Geometry: final body of the model. Coordinates: model frame, mm. Coordinates: 2 decimals unless noted, no trailing zeros. Write each loop counter-clockwise with the first axis right and the second up, starting at its lowest first coordinate (ties: lowest second). Pieces come first, ordered by that corner, then holes.
Autodesk Inventor part; units mm, degrees
ref_plane "YZ Plane" through (0, 0, 0) normal (1, 0, 0) x (0, 1, 0)
ref_plane "XZ Plane" through (0, 0, 0) normal (0, 1, 0) x (-1, 0, 0)
ref_plane "XY Plane" through (0, 0, 0) normal (0, 0, 1) x (1, 0, 0)
sketch "スケッチ1" plane through (0, 0, 0) normal (1, 0, 0) x (0, 1, 0)
  circle A0 centre (0, 0) radius 12
  line L0 (12, 0) -> (-12, 0)
  line L1 (-12, 0) -> (-12, -70)
  line L2 (-12, -70) -> (12, -70)
  line L3 (12, -70) -> (12, 0)
  line L4 (-12, -70) -> (-42, -70)
  line L5 (-42, -70) -> (-42, -46)
  line L6 (-42, -46) -> (-12, -46)
  line L7 (-12, -46) -> (-12, -70)
  point P0 (-12, -46)
  dimension "d0" = 24
  dimension "d1" = 70
  dimension "d4" = 24
  dimension "d5" = 30
extrude "押し出し1" add sketch "スケッチ1" along normal blind 5
fillet "フィレット1" radius 20 1 edges at (2.5, -12, -46)
fillet "フィレット3" radius 40 1 edges at (2.5, 12, -70)
fillet "フィレット2" radius 12 2 edges at (2.5, -42, -46) (2.5, -42, -70)
sketch "スケッチ2" plane through (5, 0, 0) normal (1, 0, 0) x (0, 0, -1)
  circle A0 centre (0, 0) radius 8.5
  point P0 (0, 8.5)
  dimension "d8" = 17
hole "穴1" at (5, 8.5, 0) direction (-1, 0, 0) diameter 3.4 end through all
pattern_circular "円形状パターン1" count 4 over 360 about axis through (0, 0, 0) along (1, 0, 0) of "穴1"
fillet "フィレット4" radius 1 16 edges at (5, -29, -70) (5, -38.4853, -66.4853) (5, -42, -57.9687) (5, -38.7464, -49.7216) (5, -12, -13) (5, 0, 12) (5, 12, -15) (5, 0.2843, -58.2843) (0, 12, -15) (0, 0, 12) (0, -12, -13) (0, -38.7464, -49.7216) (0, -42, -57.9687) (0, -38.4853, -66.4853) (0, -29, -70) (0, 0.2843, -58.2843)
properties part number "base9"
Item 1: Material intervals for probe 1 along Y at (x, z) = (1.9, 0); probe 2 along Z at (x, y) = (4.55, 0); probe 3 along Z at (x, y) = (2.55, 8.5), sorted ascending.
Derived:
probe 1: y = -12 to -10.2, -6.8 to 6.8, 10.2 to 12
probe 2: z = -58.33 to -10.2, -6.8 to 6.8, 10.2 to 11.84
probe 3: z = -46.36 to -1.7, 1.7 to 8.47
Item 2: Section A-A, the plane z = -8.5. Output: boundary loops of the cut face in (x, y).
Derived:
outline: (0, -11) arc R1 ccw to (1, -12) - (4, -12) arc R1 ccw to (5, -11) - (5, -1.7) - (0, -1.7) - close; (0, 1.7) - (5, 1.7) - (5, 11) arc R1 ccw to (4, 12) - (1, 12) arc R1 ccw to (0, 11) - close
Item 3: Section B-B, the plane x = 2.75. State how many separate pieces and enclosed holes the cut face has, plus the area to 3 significant figures.
Derived:
separate pieces: 1
enclosed holes: 4
area: 2,270 mm2
Item 4: Pin query (flat end, axial travel): pin 1 (1 mm diameter, centred on x = 4.5, y = -24.5, fed in from -Z); pin 2 (3 mm diameter, centred on x = 1.5, y = -29, fed in from +Z); pin 3 (1 mm diameter, centred on x = 2.5, y = -27.5, fed in from +Z); pin 4 (4.5 mm diameter, centred on y = 8.5, z = 0, fed in from -X). Return the tip coordinate at first contact, or that it passes through.
Derived:
pin 1: stops at z = -69.87
pin 2: stops at z = -45.49
pin 3: stops at z = -45.36
pin 4: stops at x = 0
Item 5: Pull-direction query (Y, two-part tool) for faces 1 (the flat face through (0, -10, -37)), 2 (the flat face through (2, -12, -13)), 3 (the cylindrical face through (2.46, -10.16, -0.37)); classes: released by +Y, released by -Y, zero draft, split by the parting line, or undercut.
Derived:
face 1: zero draft
face 2: released by -Y
face 3: undercut
